Geometry: see drawing. Coordinates: mm, zero at the bounding-box minimum. A direction names the side the tool comes from. Give positions to 0.01 mm unless a question says otherwise; leave off trailing zeros. Write each loop counter-clockwise with the first axis right and the second up, starting at its lowest first coordinate (ties: lowest second). Pieces come first, ordered by that corner, then holes. Notation, with made-up numbers: M 87,-19 L 135,-19 A11 ccw 135,-11 Z; hole C -13.5,69.5 d8. An arc over 180 degrees is marked long. Use a Markdown table: item, result. Add a question column.
1) Section A-A on z = 9.75. Return the cut outline in (x, y), then the cut area to 3 significant figures.
2) Section C-C on x = 5.5. Return the cut outline in (y, z), then the cut area to 3 significant figures.
3) Section D-D on z = 3.25. Return the cut outline in (x, y), then the cut area to 3 significant figures.
4) Section B-B on y = 8.25. Return the cut outline in (x, z), then the cut area to 3 significant figures.
5) Line query: line 1 (X direction, y = 2, z = 13.75); line 2 (Z direction, x = 26, y = 3); line 3 (Y direction, x = 12, z = 4.75). Output: solid intervals per line, ascending.
6) Pin query (flat end, axial travel): pin 1 (3 mm diameter, centred on x = 10, z = 13, fed in from +Y). Return the tip coordinate at first contact, or that it passes through.
7) Draft query along Z for the marked faces 3, 4, 5 and 6. Return one class per face: +Z half, -Z half, draft (parallel to the pull), parting line (faces both ways), or undercut.
8) Set-up query: the marked faces 1 and 2. Return all of +Z, -Z, +X, -X, +Y, -Y with unobstructed straight access to the full face (end or side cutting, diameter ignored); none if empty.
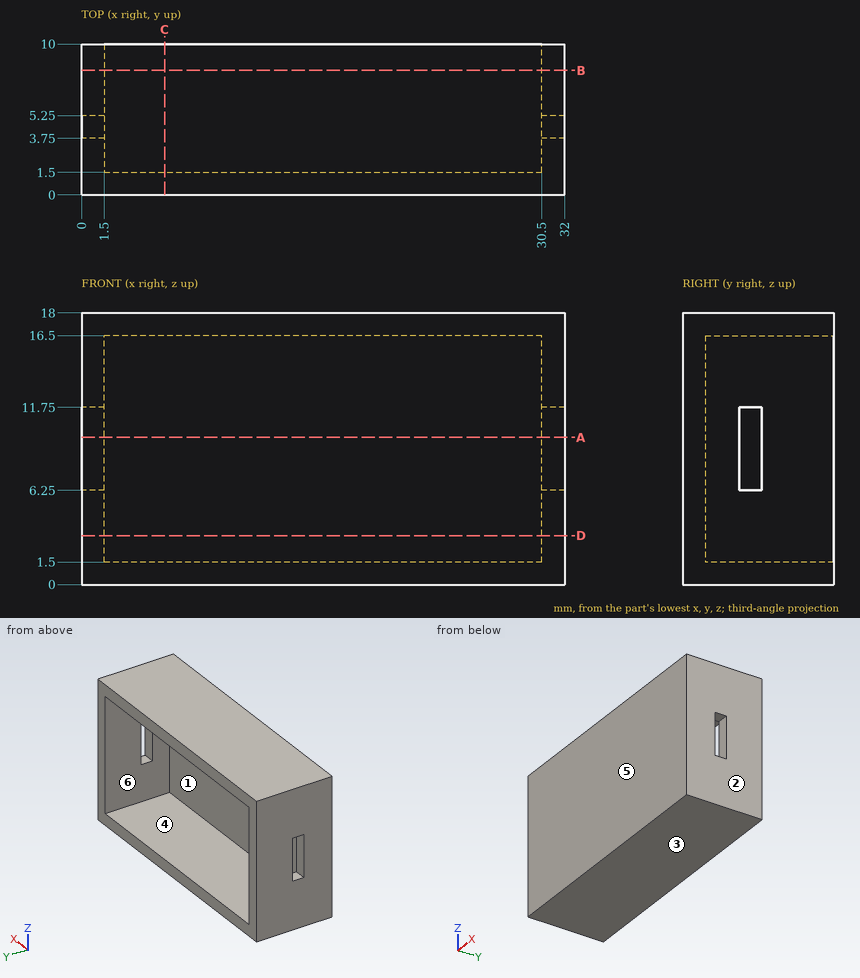
Found:
| question | item | result |
|---|---|---|
| 1 | outline | M 0,0 L 32,0 L 32,3.75 L 30.5,3.75 L 30.5,1.5 L 1.5,1.5 L 1.5,3.75 L 0,3.75 Z; M 0,5.25 L 1.5,5.25 L 1.5,10 L 0,10 Z; M 30.5,5.25 L 32,5.25 L 32,10 L 30.5,10 Z |
| 1 | area | 69.0 mm² |
| 2 | outline | M 0,0 L 10,0 L 10,1.5 L 1.5,1.5 L 1.5,16.5 L 10,16.5 L 10,18 L 0,18 Z |
| 2 | area | 52.5 mm² |
| 3 | outline | M 0,0 L 32,0 L 32,10 L 30.5,10 L 30.5,1.5 L 1.5,1.5 L 1.5,10 L 0,10 Z |
| 3 | area | 73.5 mm² |
| 4 | outline | M 0,0 L 32,0 L 32,18 L 0,18 Z; hole M 1.5,1.5 L 30.5,1.5 L 30.5,16.5 L 1.5,16.5 Z |
| 4 | area | 141 mm² |
| 5 | line 1 | 0 to 1.5, 30.5 to 32 |
| 5 | line 2 | 0 to 1.5, 16.5 to 18 |
| 5 | line 3 | 0 to 1.5 |
| 6 | pin 1 | y = 1.5 |
| 7 | face 3 | -Z half |
| 7 | face 4 | undercut |
| 7 | face 5 | draft |
| 7 | face 6 | undercut |
| 8 | face 1 | +Y |
| 8 | face 2 | +Z, -Z, +X, +Y, -Y |
